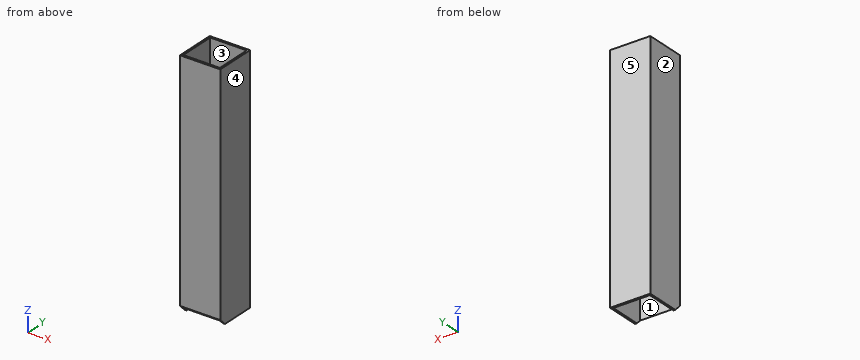
from build123d import *

# Parameters (mm, degrees)
F0_W        = 63.5
F0_H        = 63.5
F0_W_2      = 57.5
F0_H_2      = 57.5
F1_DEPTH    = 372
F2_T1_DEPTH = 114.9336597593


# Not quite as in the source:
# - a fillet or chamfer that OpenCascade refuses, or shapes differently, is made with other operations: its cross-section is extruded or revolved along the edge and cut away or added


with BuildPart() as f1:
    # F0 (on Top) → F1 (new body)
    with BuildSketch(Plane.XY):
        with Locations((4.6706348658, 6.1677011834)):
            Rectangle(F0_W, F0_H)
        with Locations((4.6706348658, 6.1677011834)):
            Rectangle(F0_W_2, F0_H_2, mode=Mode.SUBTRACT)
    extrude(amount=F1_DEPTH)

    # F2: chamfer of 10 on 1 edges, made by hand

    # F2_s2 → F2_t1 (cut)
    with BuildSketch(Plane.YZ.offset(-52.7961950139)):
        Polygon((-25.5822988166, 10), (-15.5822988166, 0), (-25.5822988166, 0), align=None)
    extrude(amount=F2_T1_DEPTH, mode=Mode.SUBTRACT)


solid = f1.part
Geometry: final body of the model. Coordinates: model frame, mm. Face numbers are marked on the shaded views. A direction names the side the tool comes from. Give positions to 0.01 mm unless a question says otherwise; leave off trailing zeros. Loops run counter-clockwise (first coordinate to the right, second up) from the corner with the lowest first, then second, coordinate; pieces in that order, holes last. Notation, with made-up numbers: (65, 7.25) -> (99, 7.25) arc R20 ccw to (99, 42.25) -> close; hole circle Ø6 at (84, -29). An arc over 180 degrees is marked (long way). Put each result on its own line as item: value.
1. Cut plane C-C (y = 18). Return the cut outline in (x, z), plus the area to 3 significant figures.
Taken from the geometry:
outline: (-27.08, 0) -> (-24.08, 0) -> (-24.08, 372) -> (-27.08, 372) -> close; (33.42, 0) -> (36.42, 0) -> (36.42, 372) -> (33.42, 372) -> close
area: 2,230 mm2
2. Ray query, line 1 along X through (y, z) = (17.5, 317); line 2 along Y through (x, z) = (-2, 165.5). Return the intervals inside material, ascending. Write a range as [from, to].
Taken from the geometry:
line 1: x = [-27.08, -24.08], [33.42, 36.42]
line 2: y = [-25.58, -22.58], [34.92, 37.92]
3. Pin query (flat end, axial travel): P1, Ø8, axis at x = 1, y = 27.5, coming from the -Z side. Return the tip coordinate at first contact, or that it passes through.
Taken from the geometry:
P1: passes through
4. Cut plane A-A (x = 28). Return the cut outline in (y, z), plus the area to 3 significant figures.
Taken from the geometry:
outline: (-25.58, 10) -> (-22.58, 7) -> (-22.58, 372) -> (-25.58, 372) -> close; (34.92, 0) -> (37.92, 0) -> (37.92, 372) -> (34.92, 372) -> close
area: 2,210 mm2
5. Cut plane B-B (z = 326). Return the cut outline in (x, y), plus the area to 3 significant figures.
Taken from the geometry:
outline: (-27.08, -25.58) -> (36.42, -25.58) -> (36.42, 37.92) -> (-27.08, 37.92) -> close; hole (-24.08, -22.58) -> (33.42, -22.58) -> (33.42, 34.92) -> (-24.08, 34.92) -> close
area: 726 mm2
6. Pull-direction query (Y, two-part tool) for the marked faces 3, 4 and 5; classes: released by +Y, released by -Y, zero draft, split by the parting line, or undercut.
Taken from the geometry:
face 3: undercut
face 4: zero draft
face 5: released by +Y
7. Set-up query: the marked faces 1 and 2. Return all of +Z, -Z, +X, -X, +Y, -Y with unobstructed straight access to the full face (end or side cutting, diameter ignored); none if empty.
Taken from the geometry:
face 1: +Z, -Z
face 2: +Z, -Z, -X, +Y, -Y
